from build123d import *

# Parameters (mm, degrees)
EXTRUDE_THIN1_START       = -406.4
EXTRUDE_THIN1_DEPTH       = 438.15
EXTRUDE_THIN1_START_2     = 13.470384182
EXTRUDE_THIN1_2_OUTLINE_W = 39
EXTRUDE_THIN1_2_OUTLINE_H = 54
EXTRUDE_THIN1_2_DEPTH     = 18.529615818
CUT_EXTRUDE2_REACH        = 409.984
CUT_EXTRUDE4_REACH        = 409.984
SKETCH5_R                 = 2.5527
CUT_EXTRUDE3_DEPTH        = 1.651
F_1_4_CLEARANCE_HOLE1_D   = 6.7564


with BuildPart() as part:
    # Extrude-Thin1: read off the stored shape, not the designer's step
    # Extrude-Thin1 outline → Extrude-Thin1 (new body)
    with BuildSketch(Plane.XY.offset(EXTRUDE_THIN1_START)):
        with BuildLine():
            ThreePointArc((-12.7, -22.86), (-11.956051224, -24.656051224), (-10.16, -25.4))
            Line((-10.16, -25.4), (10.16, -25.4))
            ThreePointArc((10.16, -25.4), (11.956051224, -24.656051224), (12.7, -22.86))
            Line((12.7, -22.86), (12.7, 22.86))
            ThreePointArc((12.7, 22.86), (11.956051224, 24.656051224), (10.16, 25.4))
            Line((10.16, 25.4), (-10.16, 25.4))
            ThreePointArc((-10.16, 25.4), (-11.956051224, 24.656051224), (-12.7, 22.86))
            Line((-12.7, 22.86), (-12.7, -22.86))
        make_face()
        with BuildLine():
            Line((10.16, -23.749), (-10.16, -23.749))
            ThreePointArc((-10.16, -23.749), (-10.788617928, -23.488617928), (-11.049, -22.86))
            Line((-11.049, -22.86), (-11.049, 22.86))
            ThreePointArc((-11.049, 22.86), (-10.788617928, 23.488617928), (-10.16, 23.749))
            Line((-10.16, 23.749), (10.16, 23.749))
            ThreePointArc((10.16, 23.749), (10.788617928, 23.488617928), (11.049, 22.86))
            Line((11.049, 22.86), (11.049, -22.86))
            ThreePointArc((11.049, -22.86), (10.788617928, -23.488617928), (10.16, -23.749))
        make_face(mode=Mode.SUBTRACT)
    extrude(amount=EXTRUDE_THIN1_DEPTH)

    # Extrude-Thin1 2 outline → Extrude-Thin1 2 (cut)
    with BuildSketch(Plane(origin=(0, 0, 0), x_dir=(0.707106781186548, 0, -0.707106781186547), z_dir=(0.707106781186547, 0, 0.707106781186548)).offset(EXTRUDE_THIN1_START_2)):
        with Locations((-13.5, 0)):
            Rectangle(EXTRUDE_THIN1_2_OUTLINE_W, EXTRUDE_THIN1_2_OUTLINE_H)
    extrude(amount=EXTRUDE_THIN1_2_DEPTH, mode=Mode.SUBTRACT)

    # Sketch3 → Cut-Extrude2 (cut, up to next)
    with BuildSketch(Plane.ZY.offset(12.7), mode=Mode.PRIVATE) as cut_extrude2_sk1:
        with BuildLine():
            Line((8.345953821, -6.6675), (-152.204543073, -6.6675))
            ThreePointArc((-152.204543073, -6.6675), (-158.872043073, 0), (-152.204543073, 6.6675))
            Line((-152.204543073, 6.6675), (8.345953821, 6.6675))
            ThreePointArc((8.345953821, 6.6675), (15.013453821, 0), (8.345953821, -6.6675))
        make_face()
    cut_extrude2_tool1 = extrude(cut_extrude2_sk1.sketch, amount=-CUT_EXTRUDE2_REACH, mode=Mode.PRIVATE) & part.part
    add(cut_extrude2_tool1.solids().sort_by_distance((-12.7, 0, -71.929295))[0], mode=Mode.SUBTRACT)

    # Sketch6 → Cut-Extrude4 (cut, up to next)
    with BuildSketch(Plane(origin=(12.7, 0, 0), x_dir=(0, 0, -1), z_dir=(1, 0, 0)), mode=Mode.PRIVATE) as cut_extrude4_sk1:
        with BuildLine():
            Line((114.104543073, 6.35), (152.204543073, 6.35))
            ThreePointArc((152.204543073, 6.35), (158.554543073, 0), (152.204543073, -6.35))
            Line((152.204543073, -6.35), (114.104543073, -6.35))
            ThreePointArc((114.104543073, -6.35), (107.754543073, 0), (114.104543073, 6.35))
        make_face()
    cut_extrude4_tool1 = extrude(cut_extrude4_sk1.sketch, amount=-CUT_EXTRUDE4_REACH, mode=Mode.PRIVATE) & part.part
    add(cut_extrude4_tool1.solids().sort_by_distance((12.7, 0, -133.154543))[0], mode=Mode.SUBTRACT)

    # Sketch5 → Cut-Extrude3 (cut)
    with BuildSketch(Plane(origin=(-12.7, 0, 0), x_dir=(0, 0, -1), z_dir=(1, 0, 0))):
        with Locations((-13.795705431, 13.589)):
            Circle(SKETCH5_R)
        with Locations((-13.795705431, -13.589)):
            Circle(SKETCH5_R)
        with Locations((71.929294569, -13.589)):
            Circle(SKETCH5_R)
        with Locations((71.929294569, 13.589)):
            Circle(SKETCH5_R)
        with Locations((157.654294569, 13.589)):
            Circle(SKETCH5_R)
        with Locations((157.654294569, -13.589)):
            Circle(SKETCH5_R)
    extrude(amount=CUT_EXTRUDE3_DEPTH, mode=Mode.SUBTRACT)

    # 1/4 Clearance Hole1 (through all)
    with Locations(Plane(origin=(0, 25.4, 0), x_dir=(1, 0, 0), z_dir=(0, 1, 0))):
        with Locations((0, 346.075), (0, 330.2), (0, 314.325), (0, 60.325), (0, 76.2), (0, 92.075)):
            Hole(F_1_4_CLEARANCE_HOLE1_D / 2)


solid = part.part
Could you check a few things on this model? Use its own coordinates, in mm. A direction names the side the tool comes from. Coordinates: 2 decimals unless noted, no trailing zeros. Order: outer loops, then holes, each group sorted by start corner. A loop starts at its lowest first (then second) coordinate and runs counter-clockwise, first axis right, second up.
Q1. Suppose I cut it at A-A on z = -191. Please give me the cut outline in (x, y).
Q2. Suppose I cut it at D-D on z = -52. Please give me the cut outline in (x, y).
Q3. Which directions (+Z, -Z, +X, -X, +Y, -Y) give clear straight access to the entire face, cutting with the end or side of a thin tool? Please do faces 4 (the flat face through (-11.049, 0, -191)), 5 (the cylindrical face through (0.732, 24.563, -57.027)), 6 (the cylindrical face through (-11.89, -0.15, -158.87)).
Q4. Suppose I cut it at C-C on z = -138.5. Please give me the cut outline in (x, y), and give its area (3 significant figures).
Q5. Thinking about a two-plate mould opening in Y: for faces 1 (the cylindrical face through (-11.89, 0.15, 15.01)), 2 (the flat face through (0, -25.4, -192)), 3 (the cylindrical face through (-1.559, 24.563, -73.203)), which applies, released by +Y, released by -Y, zero draft, split by the parting line, or undercut?
Q6. Please list where these lines run through material, in increasing order: L1, parallel to Y at x = -7.5, z = -300.5; L2, parallel to X at y = -3, z = -222.5; L3, parallel to Y at x = -10.75, z = -272.5 (3 decimals).
Q7. Will these pins go through, and if not, where does the flat tip stop? pin 1 (8 mm diameter, centred on x = -9, y = -2.5, fed in from -Z); pin 2 (6 mm diameter, centred on x = 0, z = -346.075, fed in from -Y); pin 3 (8 mm diameter, centred on y = 13.59, z = 13.8, fed in from +X); pin 4 (0.5 mm diameter, centred on x = -12, z = -80, fed in from -Y).
Q8. Suppose I cut it at B-B on y = 0. Please give me the cut outline in (x, z).
Answer:
1. outline: (-12.7, -22.86) arc R2.54 ccw to (-10.16, -25.4) - (10.16, -25.4) arc R2.54 ccw to (12.7, -22.86) - (12.7, 22.86) arc R2.54 ccw to (10.16, 25.4) - (-10.16, 25.4) arc R2.54 ccw to (-12.7, 22.86) - close; hole (-11.05, -22.86) arc R0.89 ccw to (-10.16, -23.75) - (10.16, -23.75) arc R0.89 ccw to (11.05, -22.86) - (11.05, 22.86) arc R0.89 ccw to (10.16, 23.75) - (-10.16, 23.75) arc R0.89 ccw to (-11.05, 22.86) - close
2. outline: (-12.7, -22.86) arc R2.54 ccw to (-10.16, -25.4) - (10.16, -25.4) arc R2.54 ccw to (12.7, -22.86) - (12.7, 22.86) arc R2.54 ccw to (10.16, 25.4) - (-10.16, 25.4) arc R2.54 ccw to (-12.7, 22.86) - (-12.7, 6.67) - (-11.05, 6.67) - (-11.05, 22.86) arc R0.89 cw to (-10.16, 23.75) - (10.16, 23.75) arc R0.89 cw to (11.05, 22.86) - (11.05, -22.86) arc R0.89 cw to (10.16, -23.75) - (-10.16, -23.75) arc R0.89 cw to (-11.05, -22.86) - (-11.05, -6.67) - (-12.7, -6.67) - close
3. face 4: +Z, -Z
3. face 5: +Y, -Y
3. face 6: -X
4. outline: (-12.7, -22.86) arc R2.54 ccw to (-10.16, -25.4) - (10.16, -25.4) arc R2.54 ccw to (12.7, -22.86) - (12.7, -6.35) - (11.05, -6.35) - (11.05, -22.86) arc R0.89 cw to (10.16, -23.75) - (-10.16, -23.75) arc R0.89 cw to (-11.05, -22.86) - (-11.05, -6.67) - (-12.7, -6.67) - close; (-12.7, 6.67) - (-11.05, 6.67) - (-11.05, 22.86) arc R0.89 cw to (-10.16, 23.75) - (10.16, 23.75) arc R0.89 cw to (11.05, 22.86) - (11.05, 6.35) - (12.7, 6.35) - (12.7, 22.86) arc R2.54 ccw to (10.16, 25.4) - (-10.16, 25.4) arc R2.54 ccw to (-12.7, 22.86) - close
4. area: 193 mm2
5. face 1: undercut
5. face 2: released by -Y
5. face 3: zero draft
6. L1: y = -25.4 to -23.75, 23.75 to 25.4
6. L2: x = -12.7 to -11.05, 11.05 to 12.7
6. L3: y = -25.331 to -23.525, 23.525 to 25.331
7. pin 1: stops at z = -406.4
7. pin 2: passes through
7. pin 3: stops at x = -11.05
7. pin 4: stops at y = -24.84
8. outline: (-12.7, -406.4) - (-11.05, -406.4) - (-11.05, -158.87) - (-12.7, -158.87) - close; (-12.7, 15.01) - (-11.05, 15.01) - (-11.05, 30.1) - (-12.7, 31.75) - close; (11.05, -406.4) - (12.7, -406.4) - (12.7, -158.55) - (11.05, -158.55) - close; (11.05, -107.75) - (12.7, -107.75) - (12.7, 6.35) - (11.05, 8) - close
